Check sheet for the modelled part. Datum: model origin and axes. Units: mm. Face numbers are marked on the shaded views. A direction names the side the tool comes from. Round coordinates to 2 decimals unless told otherwise and drop trailing zeros. Order: outer loops, then holes, each group sorted by start corner. A loop starts at its lowest first (then second) coordinate and runs counter-clockwise, first axis right, second up. Notation, with made-up numbers: (-23.5, 56.25) -> (-18.5, 56.25) arc R26 cw to (-18.5, 70.25) -> close; hole circle Ø2 at (-8.75, 80.5). An arc over 180 degrees is marked (long way). Answer as CSV lines item,"result". Start each with the question number.
from build123d import *

# Parameters (mm, degrees)
SKETCH1_R           = 1.6
BOSS_EXTRUDE1_DEPTH = 1.6
SKETCH2_W           = 8.2
SKETCH2_H           = 6
BOSS_EXTRUDE2_DEPTH = 2.4
SKETCH3_R           = 0.7
CUT_EXTRUDE1_DEPTH  = 6
BOSS_EXTRUDE3_DEPTH = 3.6
SKETCH5_W           = 6.1
SKETCH5_H           = 1.8
BOSS_EXTRUDE4_DEPTH = 9.2
BOSS_EXTRUDE5_DEPTH = 1.8
SKETCH7_R           = 1.6
CUT_EXTRUDE2_DEPTH  = 1.8
FILLET1_R           = 20


with BuildPart() as part:
    # Sketch1 → Boss-Extrude1 (new body)
    with BuildSketch(Plane(origin=(0, 0, 0), x_dir=(1, 0, 0), z_dir=(0, 1, 0))):
        with BuildLine():
            Line((-13.686930091, -1.927431611), (14.813069909, -1.927431611))
            ThreePointArc((14.813069909, -1.927431611), (20.913069909, 4.172568389), (14.813069909, 10.272568389))
            Line((14.813069909, 10.272568389), (6.020069909, 10.272568389))
            ThreePointArc((6.020069909, 10.272568389), (1.970069909, 6.222568389), (-2.079930091, 10.272568389))
            Line((-2.079930091, 10.272568389), (-10.686930091, 10.272568389))
            ThreePointArc((-10.686930091, 10.272568389), (-12.808250435, 9.393888733), (-13.686930091, 7.272568389))
            Line((-13.686930091, 7.272568389), (-13.686930091, 4.172568389))
            Line((-13.686930091, 4.172568389), (-13.686930091, -1.927431611))
        make_face()
        with Locations(Location((14.813069909, 4.172568389, 0), (0, 0, 270))):
            Circle(SKETCH1_R, mode=Mode.SUBTRACT)
    extrude(amount=BOSS_EXTRUDE1_DEPTH)

    # Sketch2 → Boss-Extrude2 (add)
    with BuildSketch(Plane(origin=(0, 1.6, 0), x_dir=(1, 0, 0), z_dir=(0, 1, 0))):
        with Locations((-9.586930091, 1.072568389)):
            Rectangle(SKETCH2_W, SKETCH2_H)
    extrude(amount=BOSS_EXTRUDE2_DEPTH)

    # Sketch3 → Cut-Extrude1 (cut)
    with BuildSketch(Plane.XY.offset(1.927431611)):
        with Locations((-11.585711123, 2.899970269)):
            Circle(SKETCH3_R)
        with Locations((-7.486930091, 2.8)):
            Circle(SKETCH3_R)
    extrude(amount=-CUT_EXTRUDE1_DEPTH, mode=Mode.SUBTRACT)



with BuildPart() as body_2:
    # Sketch4 → Boss-Extrude3 (new body)
    with BuildSketch(Plane.XZ):
        with BuildLine():
            Line((-13.686930091, 1.927431611), (-13.686930091, -4.172568389))
            Line((-13.686930091, -4.172568389), (-19.786930091, -4.172568389))
            ThreePointArc((-19.786930091, -4.172568389), (-18.000281456, 0.140782976), (-13.686930091, 1.927431611))
        make_face()
    extrude(amount=-BOSS_EXTRUDE3_DEPTH)


with BuildPart() as part_1:
    add(part.part)

    add(body_2.part)  # Boss-Extrude4 merges body 2
    # Sketch5 → Boss-Extrude4 (add)
    with BuildSketch(Plane(origin=(0, 0, -4.172568389), x_dir=(-1, 0, 0), z_dir=(0, 0, -1))):
        with Locations((16.736930091, 2.7)):
            Rectangle(SKETCH5_W, SKETCH5_H)
    extrude(amount=BOSS_EXTRUDE4_DEPTH)

    # Sketch6 → Boss-Extrude5 (add)
    with BuildSketch(Plane(origin=(0, 3.6, 0), x_dir=(1, 0, 0), z_dir=(0, 1, 0))):
        with BuildLine():
            Line((-19.786930091, 13.372568389), (-13.686930091, 13.372568389))
            ThreePointArc((-13.686930091, 13.372568389), (-16.736930091, 16.422568389), (-19.786930091, 13.372568389))
        make_face()
    extrude(amount=-BOSS_EXTRUDE5_DEPTH)

    # Sketch7 → Cut-Extrude2 (cut)
    with BuildSketch(Plane(origin=(0, 3.6, 0), x_dir=(1, 0, 0), z_dir=(0, 1, 0))):
        with Locations(Location((-16.530026975, 11.280054915, 0), (0, 0, 270))):
            Circle(SKETCH7_R)
    extrude(amount=-CUT_EXTRUDE2_DEPTH, mode=Mode.SUBTRACT)

    # Fillet1
    # the kernel refuses this fillet: 20 mm, written as the material it takes off along each edge
    with BuildSketch(Plane(origin=(6.020069909, -21.9825, -10.272568389), x_dir=(-0.47127431381884255, 0, 0.8819866898851587), z_dir=(0, 1, 0))) as fillet1_piece_1:
        with BuildLine():
            CenterArc((13.242808218, 17.639733798), FILLET1_R, 209.618411235, 32.264541926)
            Line((-4.143915041, 7.755308964), (-4.491649507, 7.557620467))
            ThreePointArc((-4.491649507, 7.557620467), (-2.424752197, 3.689144757), (-0.352794676, -0.188509726))
            Line((-0.352794676, -0.188509726), (0.188509726, -0.352794676))
            ThreePointArc((0.188509726, -0.352794676), (1.908660971, 0.077953906), (3.628812216, -0.352794676))
            Line((3.628812216, -0.352794676), (3.817321942, 0))
        make_face()
    extrude(amount=45.565, mode=Mode.SUBTRACT)


solid = part_1.part
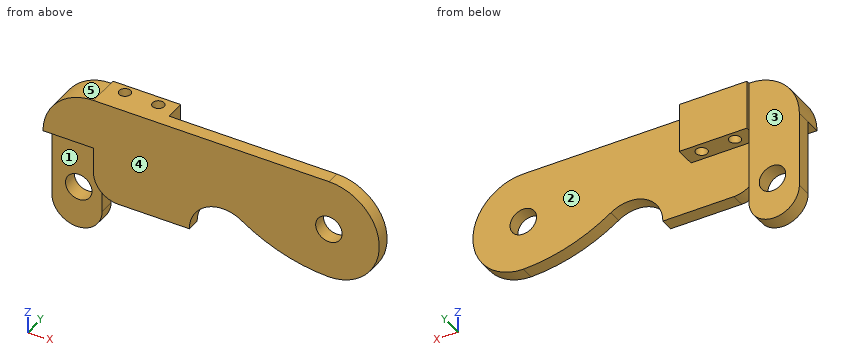
1) Section check B-B on z = -8.5. Record the cut outline in (x, y).
2) Material ranges on line 1 along X through (y, z) = (3.05, -3.5); line 2 along X through (y, z) = (3.75, 0.5); line 3 along Y through (x, z) = (16.5, 1), recorded low to high.
3) Depth check by flat-ended pin: pin 1 Ø1.2 at (x, y) = (-10.5, 3) entering from -Z; pin 2 Ø5 at (x, z) = (-16.5, -12) entering from -Y; pin 3 Ø0.6 at (y, z) = (2.5, -11) entering from +X; pin 4 Ø1.5 at (x, z) = (13.5, -3) entering from -Y. Enter the tip coordinate at first touch or a pass-through.
4) Access from +Z, -Z, +X, -X, +Y, -Y to the whole of each face (thin tool, end or side, straight path). Record for the marked faces 1, 2, 3, 4 and 5.
5) Section check C-C on z = -12. Record the cut outline in (x, y), then the cut area to 3 significant figures.
6) Section check D-D on x = 14. Record the cut outline in (y, z), then the cut area to 3 significant figures.
7) Section check A-A on x = -11.5. Record the cut outline in (y, z).
Solutions:
1,outline,"(-19.79, 1.8) -> (-13.69, 1.8) -> (-13.69, 3.6) -> (-19.79, 3.6) -> close; (-13.42, 0) -> (-1.67, 0) -> (-1.67, 1.6) -> (-13.42, 1.6) -> close; (7.09, 0) -> (19.11, 0) -> (19.11, 1.6) -> (7.09, 1.6) -> close"
2,line 1,"x = -19.75 to -12.27, -10.9 to -8.14, -6.83 to -5.49"
2,line 2,"x = -13.69 to -5.49"
2,line 3,"y = 0 to 1.6"
3,pin 1,"stops at z = -4.07"
3,pin 2,"stops at y = 1.8"
3,pin 3,"stops at x = -13.69"
3,pin 4,"stops at y = 0"
4,face 1,"-Z, +X, -X, -Y"
4,face 2,"-Z, +X, +Y"
4,face 3,"+Z, -Z, -X, +Y"
4,face 4,"+Z, -Z, +X, -X, -Y"
4,face 5,"+Z, -X, +Y, -Y"
5,outline,"(-19.79, 1.8) -> (-17.96, 1.8) -> (-17.96, 3.6) -> (-19.79, 3.6) -> close; (-15.1, 1.8) -> (-13.69, 1.8) -> (-13.69, 3.6) -> (-15.1, 3.6) -> close"
5,area,"5.84 mm^2"
6,outline,"(0, -10.23) -> (1.6, -10.23) -> (1.6, -5.55) -> (0, -5.55) -> close; (0, -2.79) -> (1.6, -2.79) -> (1.6, 1.93) -> (0, 1.93) -> close"
6,area,"15.0 mm^2"
7,outline,"(0, -10.16) -> (1.6, -10.16) -> (1.6, -4.07) -> (2.21, -4.07) -> (2.21, 1.93) -> (0, 1.93) -> close; (3.59, -4.07) -> (4, -4.07) -> (4, 1.93) -> (3.59, 1.93) -> close"
